Here's how the part is built. I have some questions about the finished solid (model axes, mm). Face numbers are marked on the shaded views. A direction names the side the tool comes from. Round coordinates to 2 decimals unless told otherwise and drop trailing zeros. Loops run counter-clockwise (first coordinate to the right, second up) from the corner with the lowest first, then second, coordinate; pieces in that order, holes last. Notation, with made-up numbers: M 62,65 L 84,65 A28 cw 84,89 Z; hole C 41.5,13.5 d7. An arc over 180 degrees is marked long. Answer as CSV lines item,"result".
```python
from build123d import *

# Parameters (mm, degrees)
F0_W          = 166
F0_H          = 20
F0_R          = 2.4
F1_DEPTH      = 10
F2_W          = 12
F2_H          = 14
F3_DEPTH      = 7
F5_DEPTH      = 3.001
F5_DEPTH_BACK = 17.001
F6_R          = 4
F7_R          = 1
F8_R          = 3
F9_DEPTH      = 3.001
F10_W         = 55.2
F10_H         = 12
F10_W_2       = 19.2
F11_DEPTH     = 10.001
F12_R         = 4
F13_SIZE      = 0.6


with BuildPart() as f1:
    # F0 (on Top) → F1 (new body)
    with BuildSketch(Plane.XY):
        with Locations((83, 10)):
            Rectangle(F0_W, F0_H)
        with Locations((17, 10)):
            Circle(F0_R, mode=Mode.SUBTRACT)
        with Locations((49, 10)):
            Circle(F0_R, mode=Mode.SUBTRACT)
        with Locations((117, 10)):
            Circle(F0_R, mode=Mode.SUBTRACT)
        with Locations((149, 10)):
            Circle(F0_R, mode=Mode.SUBTRACT)
    extrude(amount=F1_DEPTH)

    # F2 (on face) → F3 (cut)
    with BuildSketch(Plane.XY.offset(10)):
        with Locations((6, 10)):
            Rectangle(F2_W, F2_H)
        with Locations((160, 10)):
            Rectangle(F2_W, F2_H)
    extrude(amount=-F3_DEPTH, mode=Mode.SUBTRACT)

    # F4 (on face) → F5 (cut, two sides)
    with BuildSketch(Plane.XZ.offset(-17)) as f5_sk:
        Polygon((0, 10), (0, 3), (12, 10), align=None)
        Polygon((166, 3), (166, 10), (154, 10), align=None)
    extrude(amount=-F5_DEPTH, mode=Mode.SUBTRACT)
    extrude(f5_sk.sketch, amount=F5_DEPTH_BACK, mode=Mode.SUBTRACT)

    # F6
    f6_edges = [f1.edges().sort_by_distance(p)[0] for p in [
        (12, 17, 6.5),
        (12, 3, 6.5),
        (154, 3, 6.5),
        (154, 17, 6.5),
    ]]
    fillet(f6_edges, radius=F6_R)

    # F7
    f7_edges = [f1.edges().sort_by_distance(p)[0] for p in [
        (162, 17, 3),
        (4, 3, 3),
    ]]
    fillet(f7_edges, radius=F7_R)

    # F8 (on face) → F9 (cut, through all)
    with BuildSketch(Plane.XY.offset(3)):
        with Locations((160, 10)):
            Circle(F8_R)
        with Locations((6, 10)):
            Circle(F8_R)
    extrude(amount=-F9_DEPTH, mode=Mode.SUBTRACT)

    # F10 (on face) → F11 (cut, through all)
    with BuildSketch(Plane(origin=(0, 0, 0), x_dir=(1, 0, 0), z_dir=(0, 0, -1))):
        with Locations((83, -10)):
            Rectangle(F10_W, F10_H)
        with Locations((133, -10)):
            Rectangle(F10_W_2, F10_H)
        with Locations((33, -10)):
            Rectangle(F10_W_2, F10_H)
    extrude(amount=-F11_DEPTH, mode=Mode.SUBTRACT)

    # F12
    f12_edges = [f1.edges().sort_by_distance(p)[0] for p in [
        (123.4, 16, 5),
        (123.4, 4, 5),
        (142.6, 16, 5),
        (142.6, 4, 5),
        (110.6, 16, 5),
        (110.6, 4, 5),
        (55.4, 16, 5),
        (55.4, 4, 5),
        (42.6, 4, 5),
        (42.6, 16, 5),
        (23.4, 16, 5),
        (23.4, 4, 5),
    ]]
    fillet(f12_edges, radius=F12_R)

    # F13
    f13_edges = [f1.edges().sort_by_distance(p)[0] for p in [
        (3, 10, 3),
        (14.6, 10, 10),
        (46.6, 10, 10),
        (114.6, 10, 10),
        (146.6, 10, 10),
        (157, 10, 3),
    ]]
    chamfer(f13_edges, length=F13_SIZE)


solid = f1.part
```
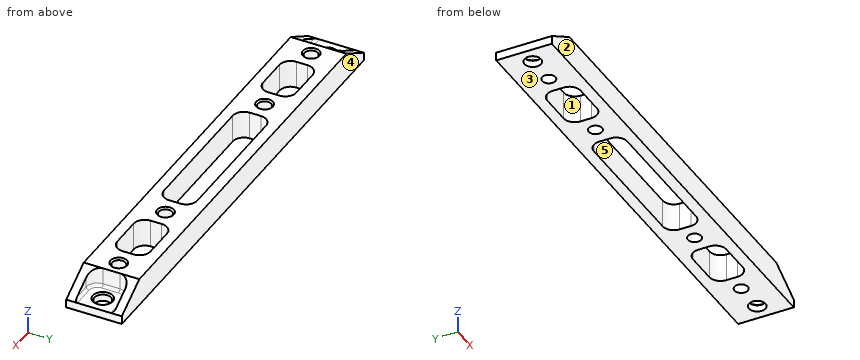
1. Which directions (+Z, -Z, +X, -X, +Y, -Y) give clear straight access to the entire face, cutting with the end or side of a thin tool? Please do the marked faces 4 and 5.
Evaluation:
face 4,"+Z, -Z, +X, -X, +Y"
face 5,"+Z, -Z"
2. I want a section at C-C, the plane y = 10. Count the separate pieces of the cut face and the enclosed holes in it, and give its area (3 significant figures).
Evaluation:
separate pieces,"10"
enclosed holes,"0"
area,"326 mm²"
3. We'd pull the mould along Y, two halves only. Please class the marked faces 1, 2 and 3: pulls with the +Y half, pulls with the -Y half, needs draft (parallel to the pull), parting line crosses it, or undercut.
Evaluation:
face 1,"undercut"
face 2,"pulls with the -Y half"
face 3,"needs draft"
4. For P1, Ø10, axis at x = 145.5, y = 2.5, coming from the -Z side; P2, Ø3, axis at y = 8.5, z = 8.5, coming from the +X side; P3, Ø1.1, axis at x = 4.5, z = 6.5, coming from the +Y side (3 decimals); P4, Ø3, axis at y = 11, z = 6, coming from the -X side, each with a flat end and sliding along its axis, tell me the tip position at first contact or that it passes through.
Evaluation:
P1,"stops at z = 0"
P2,"stops at x = 154"
P3,"passes through"
P4,"stops at x = 12"
5. If I drill on line 1 (Y direction, x = 133.5, z = 8.25); line 2 (X direction, y = 7.5, z = 5.25); line 3 (X direction, y = 6, z = 8.5), over which ranges is the centre line in solid material (lowest first)? Write a range as [from, to].
Evaluation:
line 1,"y = [0, 4], [16, 20]"
line 2,"x = [12, 23.43], [42.57, 55.43], [110.57, 123.43], [142.57, 154]"
line 3,"x = [11.87, 23.94], [42.06, 55.94], [110.06, 123.94], [142.06, 154.13]"
6. I want a section at A-A, the plane x = 117. Please give me the cut outline in (y, z), and give its area (3 significant figures).
Evaluation:
outline,"M 0,0 L 7.6,0 L 7.6,9.4 L 7,10 L 0,10 Z; M 12.4,0 L 20,0 L 20,10 L 13,10 L 12.4,9.4 Z"
area,"152 mm²"
7. I want a section at B-B, the plane x = 90. Please give me the cut outline in (y, z), and give its area (3 significant figures).
Evaluation:
outline,"M 0,0 L 4,0 L 4,10 L 0,10 Z; M 16,0 L 20,0 L 20,10 L 16,10 Z"
area,"80.0 mm²"
